Autodesk Inventor part; units mm, degrees
ref_plane "YZ Plane" through (0, 0, 0) normal (1, 0, 0) x (0, 1, 0)
ref_plane "XZ Plane" through (0, 0, 0) normal (0, 1, 0) x (-1, 0, 0)
ref_plane "XY Plane" through (0, 0, 0) normal (0, 0, 1) x (1, 0, 0)
sketch "Skizze1" plane through (0, 0, 0) normal (1, 0, 0) x (0, 1, 0)
  line L0 (-20, -20) -> (20, -20)
  line L1 (20, -20) -> (20, 20)
  line L2 (20, 20) -> (-20, 20)
  line L3 (-20, 20) -> (-20, -20)
  line L4 (-20, -20) -> (20, 20) construction
  line L5 (20, -20) -> (-20, 20) construction
  line L6 (-16, -16) -> (16, -16) construction
  line L7 (16, -16) -> (16, 16) construction
  line L8 (16, 16) -> (-16, 16) construction
  line L9 (-16, 16) -> (-16, -16) construction
  line L10 (-16, -16) -> (16, 16) construction
  line L11 (16, -16) -> (-16, 16) construction
  circle A0 centre (16, 16) radius 2.25
  circle A1 centre (16, -16) radius 2.25
  circle A2 centre (-16, -16) radius 2.25
  circle A3 centre (-16, 16) radius 2.25
  line L12 (-20, 20) -> (-32, 20)
  line L13 (-32, 20) -> (-32, -20)
  line L14 (-32, -20) -> (-20, -20)
  line L15 (-20, -20) -> (-20, 20)
  point P0 (0, 0)
  dimension "d0" = 40
  dimension "d1" = 40
  dimension "d2" = 32
  dimension "d3" = 32
  dimension "d4" = 4.5
  dimension "d5" = 4.5
  dimension "d6" = 4.5
  dimension "d7" = 4.5
  dimension "d8" = 12
extrude "Extrusion1" add sketch "Skizze1" along normal blind 6
ref_plane "Arbeitsebene1" through (0, -32, 20) normal (0, 0, 1) x (1, 0, 0)
sketch "Skizze2" plane through (0, -32, 20) normal (0, 0, 1) x (1, 0, 0)
  line L0 (0, 52) -> (0, 0)
  line L1 (0, 0) -> (6, 0)
  line L2 (6, 52) -> (6, 0)
  line L3 (0, 52) -> (6, 52)
  line L4 (-18, 6) -> (-12, 6)
  line L5 (-12, 6) -> (-12, -39)
  line L6 (-12, -39) -> (-18, -39)
  line L7 (-18, -39) -> (-18, 6)
  line L8 (0, 0) -> (-12, -6)
  line L9 (-12, 6) -> (0, 6)
  point P0 (0, 32)
  point P1 (-15, -39)
  point P2 (-15, 6)
  dimension "d12" = 6
  dimension "d13" = 45
  dimension "d14" = 6
  dimension "d15" = 12
  dimension "d16" = 12
extrude "Extrusion2" add sketch "Skizze2" against normal up to surface (40 mm away) contours L0 L8 L5 L9 | L5 L6 L7 L4
chamfer "Fasen1" distance 2 angle 45 6 edges at (-18, -26, 0) (0, -26, 0) (-15, -71, -20) (-15, -71, 20) (3, 20, -20) (3, 20, 20)
sketch "Skizze3" plane through (-12, -38, 20) normal (1, 0, 0) x (0, 0, -1)
  line L0 (2, -33) -> (0, -31)
  line L1 (2, -33) -> (38, -33)
  line L2 (40, -31) -> (38, -33)
  line L3 (40, 0) -> (40, -31)
  line L4 (0, 0) -> (40, 0)
  line L5 (0, -31) -> (0, 0)
  circle A0 centre (20, -13) radius 20
  circle A1 centre (20, -13) radius 16.5
  point P0 (20, 38)
  dimension "d22" = 33
extrude "Extrusion3" cut sketch "Skizze3" along normal through all contours A1 L4 | L4 A1
sketch "Skizze4" plane through (-12, -69, 20) normal (1, 0, 0) x (0, 0, -1)
  line L0 (0, 31) -> (9.8388, 31)
  line L1 (0, 0) -> (0, 31)
  line L2 (2, -2) -> (0, 0)
  line L3 (2, -2) -> (38, -2)
  line L4 (40, 0) -> (38, -2)
  line L5 (40, 31) -> (40, 0)
  line L6 (30.1612, 31) -> (40, 31)
  arc A0 (30.1612, 31) -> (9.8388, 31) centre (20, 18) ccw
  circle A1 centre (20, 18) radius 16.5
  circle A2 centre (3.5, 18) radius 2
  circle A3 centre (36.5, 18) radius 2
  point P0 (20, 69)
  dimension "d25" = 4
  dimension "d26" = 4
extrude "Extrusion4" cut sketch "Skizze4" against normal blind 10 contours A2 A1 | A1 A2 | A3 A1 | A1 A3
sketch "Skizze5" plane through (-12, -69, 20) normal (1, 0, 0) x (0, 0, -1)
  arc A0 (30.1612, 31) -> (9.8388, 31) centre (20, 18) ccw
  line L0 (0, 37) -> (40, 37)
  line L1 (0, 31) -> (0, 37)
  line L2 (0, 31) -> (9.8388, 31)
  circle A1 centre (20, 18) radius 11
  line L3 (30.1612, 31) -> (40, 31)
  line L4 (40, 37) -> (40, 31)
  point P0 (20, 69)
  dimension "d29" = 22
extrude "Extrusion5" cut sketch "Skizze5" against normal blind 10 contours A1
fillet "Rundung1" radius 1 1 edges at (6, -32, 0)
properties part number "40_XYZstage_micrometer_motorized_nema8_samplemount_lightsheet_screwed"
CAD build for the part. Positions are in the model's coordinates, mm. A direction names the side the tool comes from. Give positions to 0.01 mm unless a question says otherwise; leave off trailing zeros. Order: outer loops, then holes, each group sorted by start corner. A loop starts at its lowest first (then second) coordinate and runs counter-clockwise, first axis right, second up.
(1) Saw through at D-D, the plane y = -16. Give the cut face in (x, z), then the cut area to 3 significant figures.
(2) Saw through at B-B, the plane z = 2. Give the cut face in (x, y).
(3) Drill centre lines: L1, parallel to Z at x = 1.75, y = 16; L2, parallel to X at y = 16.5, z = 2; L3, parallel to Y at x = 1.5, z = -7. Where is each one in solid material? Low to high.
(4) Saw through at A-A, the plane y = -51. Give the cut face in (x, z).
(5) Flat gauge pins, fed straight in: pin 1 (4 mm diameter, centred on x = -2, z = 15, fed in from -Y); pin 2 (1.5 mm diameter, centred on x = 3.5, z = 9.5, fed in from -Y); pin 3 (4 mm diameter, centred on x = -6, z = 0.5, fed in from +Y); pin 4 (5 mm diameter, centred on x = -1.5, y = -19, fed in from -Z). Where does each tip first touch, or does it go through?
(6) Tool access for faces 1 (the cylindrical face through (2.958, -14.962, -14.004)), 2 (the flat face through (-9, -26, 0)), 3 (the cylindrical face through (-9.3, -34.5, 0.2)): list every direction of +Z, -Z, +X, -X, +Y, -Y with a clear straight run to the whole face (end or side of a thin tool).
(7) Saw through at C-C, the plane x = 4. Give the cut face in (y, z), then the cut area to 3 significant figures.
(8) Mould opens along Y. For faces 4 (the flat face through (-17, -27, 0)), 5 (the flat face through (-12, -65, 0)), 6 (the cylindrical face through (-14.958, -52.952, 16.934)) say: released by +Y, released by -Y, zero draft, split by the parting line, or undercut.
Results found:
1. outline: (0, -20) - (6, -20) - (6, -18.25) - (0, -18.25) - close; (0, -13.75) - (6, -13.75) - (6, 13.75) - (0, 13.75) - close; (0, 18.25) - (6, 18.25) - (6, 20) - (0, 20) - close
1. area: 186 mm2
2. outline: (-18, -71) - (-12, -71) - (-12, -61.82) - (-18, -61.82) - close; (-18, -40.18) - (-12, -40.18) - (-12, -34.62) - (-5.24, -34.62) - (0, -32) - (5, -32) arc R1 ccw to (6, -31) - (6, 20) - (0, 20) - (0, -24) - (-2, -26) - (-16, -26) - (-18, -28) - close
3. L1: z = -20 to -18.25, -13.75 to 13.75, 18.25 to 20
3. L2: x = 0 to 6
3. L3: y = -32 to 20
4. outline: (-18, -20) - (-12, -20) - (-12, -18.5) - (-18, -18.5) - close; (-18, -14.5) - (-12, -14.5) - (-12, -11) - (-18, -11) - close; (-18, 11) - (-12, 11) - (-12, 14.5) - (-18, 14.5) - close; (-18, 18.5) - (-12, 18.5) - (-12, 20) - (-18, 20) - close
5. pin 1: stops at y = -34
5. pin 2: stops at y = -32
5. pin 3: stops at y = -26
5. pin 4: stops at z = -20
6. face 1: +X, -X
6. face 2: +Z, -Z, -X, +Y
6. face 3: +X, -Y
7. outline: (-32, -20) - (18, -20) - (20, -18) - (20, 18) - (18, 20) - (-32, 20) - close; hole circle Ø4.5 at (-16, -16); hole circle Ø4.5 at (-16, 16); hole circle Ø4.5 at (16, -16); hole circle Ø4.5 at (16, 16)
7. area: 2,010 mm2
8. face 4: released by +Y
8. face 5: zero draft
8. face 6: undercut
